The drawing under review shows one solid part. Ordinate dimensions are in mm from its lowest x, y, z. Round coordinates to 2 decimals unless told otherwise and drop trailing zeros. Write each loop counter-clockwise with the first axis right and the second up, starting at its lowest first coordinate (ties: lowest second). Pieces come first, ordered by that corner, then holes.
Item 1: Clearance check with flat-ended pins moving along their axes: pin 1 Ø0.9 at (x, y) = (65.5, 1) entering from -Z; pin 2 Ø2.5 at (x, z) = (16, 7) entering from -Y; pin 3 Ø1.5 at (x, y) = (52, 2) entering from +Z; pin 4 Ø0.9 at (y, z) = (1, 25.5) entering from -X. State where each tip first meets the part, or that it passes through.
Item 2: Add section B-B (z = 27). Give the boundary of the cut face in (x, y), plus the area to 3 significant figures.
Item 3: To check wall thickness, follow L1, parallel to X at y = 0.95, z = 27; L2, parallel to X at y = 1.7, z = 47; L3, parallel to Z at x = 54, y = 0.65. State the ranges of each line that lie inside material, in increasing order.
Item 4: Add section A-A (x = 37). Give the boundary of the cut face in (y, z).
Item 5: Add section D-D (x = 16). Give the boundary of the cut face in (y, z).
Item 6: Add section C-C (y = 0.6). Give the boundary of the cut face in (x, z).
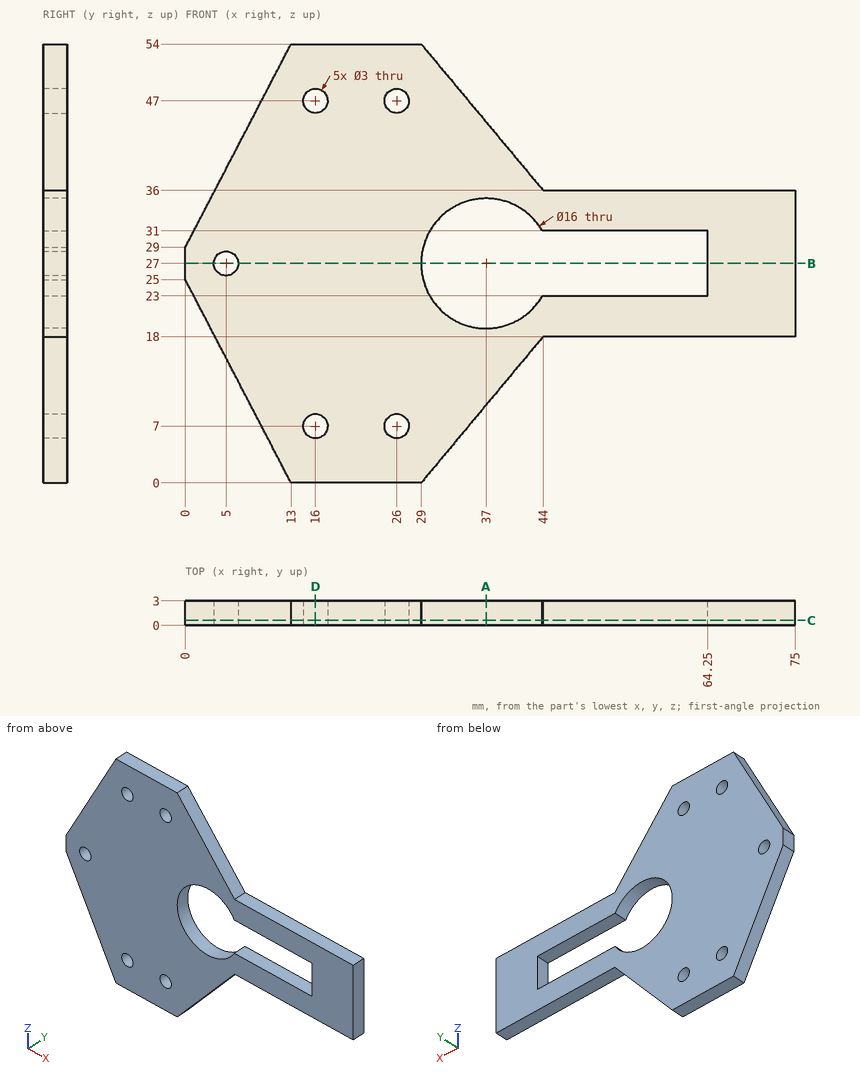
Numbers:
1. pin 1: stops at z = 18
1. pin 2: passes through
1. pin 3: stops at z = 36
1. pin 4: stops at x = 0
2. outline: (0, 0) - (3.5, 0) - (3.5, 3) - (0, 3) - close; (6.5, 0) - (29, 0) - (29, 3) - (6.5, 3) - close; (64.25, 0) - (75, 0) - (75, 3) - (64.25, 3) - close
2. area: 110 mm2
3. L1: x = 0 to 3.5, 6.5 to 29, 64.25 to 75
3. L2: x = 9.36 to 14.5, 17.5 to 24.5, 27.5 to 34.83
3. L3: z = 18 to 23, 31 to 36
4. outline: (0, 9.6) - (3, 9.6) - (3, 19) - (0, 19) - close; (0, 35) - (3, 35) - (3, 44.4) - (0, 44.4) - close
5. outline: (0, 0) - (3, 0) - (3, 5.5) - (0, 5.5) - close; (0, 8.5) - (3, 8.5) - (3, 45.5) - (0, 45.5) - close; (0, 48.5) - (3, 48.5) - (3, 54) - (0, 54) - close
6. outline: (0, 25) - (13, 0) - (29, 0) - (44, 18) - (75, 18) - (75, 36) - (44, 36) - (29, 54) - (13, 54) - (0, 29) - close; hole circle Ø3 at (5, 27); hole circle Ø3 at (16, 7); hole circle Ø3 at (16, 47); hole circle Ø3 at (26, 7); hole circle Ø3 at (26, 47); hole (43.93, 23) - (64.25, 23) - (64.25, 31) - (43.93, 31) arc R8 ccw (long way) to start
